```python
from build123d import *

# Parameters (mm, degrees)
ESBO_O1_R                  = 15
ESBO_O1_R_2                = 12.5
RESSALTO_EXTRUS_O1_DEPTH   = 210
RESSALTO_EXTRUS_O3_START   = 10
ESBO_O2_R                  = 12.5
ESBO_O2_R_2                = 10
RESSALTO_EXTRUS_O3_DEPTH   = 15
CORTE_EXTRUS_O2_DEPTH      = 300
CORTE_EXTRUS_O2_DEPTH_BACK = 300
ESBO_O4_R                  = 2.5
CORTE_EXTRUS_O3_DEPTH      = 300
CORTE_EXTRUS_O3_DEPTH_BACK = 300
ESBO_O4_3_R                = 2.5
ESBO_O6_W                  = 10
ESBO_O6_H                  = 15
CORTE_EXTRUS_O4_DEPTH      = 20


with BuildPart() as part:
    # Esbo_o1 → Ressalto-extrus_o1 (new body)
    with BuildSketch(Plane(origin=(0, 0, 0), x_dir=(0, 0, -1), z_dir=(1, 0, 0))):
        Circle(ESBO_O1_R)
        Circle(ESBO_O1_R_2, mode=Mode.SUBTRACT)
    extrude(amount=RESSALTO_EXTRUS_O1_DEPTH)

    # Esbo_o2 → Ressalto-extrus_o3 (add)
    with BuildSketch(Plane.ZY.offset(RESSALTO_EXTRUS_O3_START)):
        Circle(ESBO_O2_R)
        Circle(ESBO_O2_R_2, mode=Mode.SUBTRACT)
    extrude(amount=-RESSALTO_EXTRUS_O3_DEPTH)

    # Esbo_o4 → Corte-extrus_o2 (cut, two sides: drawn at the far end of the back side and taken through both)
    with BuildSketch(Plane(origin=(0, 0, 0), x_dir=(1, 0, 0), z_dir=(0, 1, 0)).offset(-CORTE_EXTRUS_O2_DEPTH_BACK)):
        with Locations(Location((205, 0, 0), (0, 0, 90))):
            Circle(ESBO_O4_R)
    extrude(amount=CORTE_EXTRUS_O2_DEPTH + CORTE_EXTRUS_O2_DEPTH_BACK, mode=Mode.SUBTRACT)

    # Esbo_o4_3 → Corte-extrus_o3 (cut, two sides: drawn at the far end of the back side and taken through both)
    with BuildSketch(Plane(origin=(0, 0, 0), x_dir=(1, 0, 0), z_dir=(0, 1, 0)).offset(-CORTE_EXTRUS_O3_DEPTH_BACK)):
        with Locations(Location((-5, 0.5, 0), (0, 0, 90))):
            Circle(ESBO_O4_3_R)
        with Locations(Location((205, 0, 0), (0, 0, 90))):
            Circle(ESBO_O4_3_R)
    extrude(amount=CORTE_EXTRUS_O3_DEPTH + CORTE_EXTRUS_O3_DEPTH_BACK, mode=Mode.SUBTRACT)

    # Esbo_o6 → Corte-extrus_o4 (cut)
    with BuildSketch(Plane(origin=(0, 0, 0), x_dir=(1, 0, 0), z_dir=(0, 1, 0))):
        with Locations((190, 0)):
            Rectangle(ESBO_O6_W, ESBO_O6_H)
    extrude(amount=CORTE_EXTRUS_O4_DEPTH, mode=Mode.SUBTRACT)


solid = part.part
```
Can you work these out from the model? Positions are in its coordinate system, mm. A direction names the side the tool comes from. Round coordinates to 2 decimals unless told otherwise and drop trailing zeros. Loops run counter-clockwise (first coordinate to the right, second up) from the corner with the lowest first, then second, coordinate; pieces in that order, holes last.
Item 1: Which directions (+Z, -Z, +X, -X, +Y, -Y) give clear straight access to the entire face, cutting with the end or side of a thin tool? Please do faces 1 (the cylindrical face through (-2.605, -3.83, 9.237)), 2 (the flat face through (195, 13, 0)), 3 (the cylindrical face through (-5.07, -11.09, 5.77)), 4 (the flat face through (5, 10.2, -0.1)), 5 (the cylindrical face through (-7.48, 11, -0.17)).
Item 2: Suppose I cut it at B-B, the plane z = 4.5. Write out the boundary of the cut face in (x, y).
Item 3: Please list where these lines run through material, in increasing order: L1, parallel to X at y = 13.25, z = 0; L2, parallel to X at y = 10.8, z = -0.5; L3, parallel to Z at x = 131, y = -0.5.
Item 4: Suppose I cut it at D-D, the plane x = 156. Write out the boundary of the cut face in (y, z).
Item 5: Suppose I cut it at C-C, the plane x = 205. Write out the boundary of the cut face in (y, z), then the cut area to 3 significant figures.
Item 6: Will these pins go through, and if not, where does the flat tip stop? pin 1 Ø5 at (x, z) = (101.5, 0.5) entering from +Y; pin 2 Ø3.5 at (x, y) = (190, 12) entering from -Z; pin 3 Ø12.5 at (y, z) = (5.5, -0.5) entering from +X; pin 4 Ø3.5 at (x, y) = (192, 11.5) entering from +Z.
Item 7: Suppose I cut it at A-A, the plane y = 0. Write out the boundary of the cut face in (x, z), then the cut area to 4 significant figures.
Item 8: If we mould it in two halves opening along Z, with no side actions, what happens to faces 6 (the cylindrical face through (103.53, 0.66, 14.985)), 7 (the flat face through (210, 12.3, 3.4)), 8 (the cylindrical face through (203.31, -13.64, 1.84))? For each: +Z half, -Z half, draft (parallel to the pull), parting line (faces both ways), or undercut.
Reported:
1. face 1: +X, -X
1. face 2: +Y
1. face 3: -X
1. face 4: +X
1. face 5: +Y, -Y
2. outline: (-10, -11.66) - (0, -11.66) - (0, -14.31) - (210, -14.31) - (210, -11.66) - (5, -11.66) - (5, -8.93) - (-10, -8.93) - close; (-10, 8.93) - (5, 8.93) - (5, 11.66) - (185, 11.66) - (185, 14.31) - (0, 14.31) - (0, 11.66) - (-10, 11.66) - close; (195, 11.66) - (210, 11.66) - (210, 14.31) - (195, 14.31) - close
3. L1: x = 0 to 185, 195 to 202.5, 207.5 to 210
3. L2: x = -10 to -7.5, -2.5 to 5
3. L3: z = -14.99 to -12.49, 12.49 to 14.99
4. outline: circle Ø30 at (0, 0); hole circle Ø25 at (0, 0)
5. outline: (-14.79, -2.5) arc R15 ccw to (14.79, -2.5) - (12.25, -2.5) arc R12.5 cw to (-12.25, -2.5) - close; (-14.79, 2.5) - (-12.25, 2.5) arc R12.5 cw to (12.25, 2.5) - (14.79, 2.5) arc R15 ccw to start
5. area: 191 mm2
6. pin 1: stops at y = 15
6. pin 2: stops at z = -10.95
6. pin 3: stops at x = 5
6. pin 4: stops at z = 11.4
7. outline: (-10, -12.5) - (0, -12.5) - (0, -15) - (210, -15) - (210, -12.5) - (5, -12.5) - (5, -10) - (-10, -10) - close; (-10, 10) - (5, 10) - (5, 12.5) - (210, 12.5) - (210, 15) - (0, 15) - (0, 12.5) - (-10, 12.5) - close
7. area: 1,125 mm2
8. face 6: parting line
8. face 7: draft
8. face 8: undercut
